Read the model definition and answer for the solid it produces. Units are mm, in the model's axes. Give positions to 0.01 mm unless a question says otherwise; leave off trailing zeros.
```python
from build123d import *

# Parameters (mm, degrees)
SKETCH1_W           = 476.25
SKETCH1_H           = 114.3
BOSS_EXTRUDE1_DEPTH = 6.35
SKETCH2_W           = 463.55
SKETCH2_H           = 6.35
CUT_EXTRUDE1_DEPTH  = 3.175
SKETCH2_3_W         = 463.55
SKETCH2_3_H         = 6.35
SKETCH2_3_W_2       = 469.9
SKETCH2_3_H_2       = 1.5875
CUT_EXTRUDE2_DEPTH  = 3.175


with BuildPart() as part:
    # Sketch1 → Boss-Extrude1 (new body)
    with BuildSketch(Plane(origin=(0, 0, 0), x_dir=(1, 0, 0), z_dir=(0, 1, 0))):
        with Locations((238.125, 57.15)):
            Rectangle(SKETCH1_W, SKETCH1_H)
    extrude(amount=-BOSS_EXTRUDE1_DEPTH)

    # Sketch2 → Cut-Extrude1 (cut)
    with BuildSketch(Plane(origin=(0, 0, 0), x_dir=(1, 0, 0), z_dir=(0, 1, 0))):
        with Locations((238.125, 109.855)):
            Rectangle(SKETCH2_W, SKETCH2_H)
        with BuildLine():
            ThreePointArc((6.35, 106.68), (3.175, 109.855), (6.35, 113.03))
            Line((6.35, 113.03), (6.35, 106.68))
        make_face()
        with Locations((238.125, 56.8325)):
            Rectangle(SKETCH2_W, SKETCH2_H)
        with BuildLine():
            ThreePointArc((6.35, 53.6575), (3.175, 56.8325), (6.35, 60.0075))
            Line((6.35, 60.0075), (6.35, 53.6575))
        make_face()
        with Locations((238.125, 37.7825)):
            Rectangle(SKETCH2_W, SKETCH2_H)
        with BuildLine():
            ThreePointArc((6.35, 34.6075), (3.175, 37.7825), (6.35, 40.9575))
            Line((6.35, 40.9575), (6.35, 34.6075))
        make_face()
        with BuildLine():
            ThreePointArc((6.35, 15.5575), (3.175, 18.7325), (6.35, 21.9075))
            Line((6.35, 21.9075), (6.35, 15.5575))
        make_face()
        with BuildLine():
            ThreePointArc((3.175, 1.27), (2.38125, 2.06375), (3.175, 2.8575))
            Line((3.175, 2.8575), (3.175, 1.27))
        make_face()
        with BuildLine():
            Line((469.9, 106.68), (469.9, 113.03))
            ThreePointArc((469.9, 113.03), (473.075, 109.855), (469.9, 106.68))
        make_face()
        with BuildLine():
            ThreePointArc((469.9, 60.0075), (473.075, 56.8325), (469.9, 53.6575))
            Line((469.9, 53.6575), (469.9, 60.0075))
        make_face()
        with BuildLine():
            ThreePointArc((469.9, 40.9575), (473.075, 37.7825), (469.9, 34.6075))
            Line((469.9, 34.6075), (469.9, 40.9575))
        make_face()
        with BuildLine():
            ThreePointArc((469.9, 21.9075), (473.075, 18.7325), (469.9, 15.5575))
            Line((469.9, 15.5575), (469.9, 21.9075))
        make_face()
        with BuildLine():
            ThreePointArc((473.075, 2.8575), (473.86875, 2.06375), (473.075, 1.27))
            Line((473.075, 1.27), (473.075, 2.8575))
        make_face()
    extrude(amount=-CUT_EXTRUDE1_DEPTH, mode=Mode.SUBTRACT)

    # Sketch2_3 → Cut-Extrude2 (cut)
    with BuildSketch(Plane(origin=(0, 0, 0), x_dir=(1, 0, 0), z_dir=(0, 1, 0))):
        with Locations((238.125, 18.7325)):
            Rectangle(SKETCH2_3_W, SKETCH2_3_H)
        with Locations((238.125, 2.06375)):
            Rectangle(SKETCH2_3_W_2, SKETCH2_3_H_2)
    extrude(amount=-CUT_EXTRUDE2_DEPTH, mode=Mode.SUBTRACT)


solid = part.part
```
1) The part is cut by section A-A on y = -1. Count the separate pieces of the cut face and the enclosed holes in it, and give its area (3 significant figures).
Final values:
separate pieces: 1
enclosed holes: 5
area: 41,800 mm2
2) Given pin 1 (3 mm diameter, centred on x = 151, z = -17.5, fed in from +Y) (3 decimals); pin 2 (1 mm diameter, centred on y = -2, z = -88.5, fed in from -X), each flat-ended and moving along its own axis, determine where each tip first touches the part or whether it passes through.
Final values:
pin 1: stops at y = -3.175
pin 2: stops at x = 0
3) Consider L1, parallel to Z at x = 246, y = -2.75; L2, parallel to X at y = -1, z = -16; L3, parallel to X at y = -1.5, z = -40. Determine where each line is inside the solid, lowest interval first.
Final values:
L1: z = -114.3 to -113.03, -106.68 to -60.01, -53.66 to -40.96, -34.61 to -21.91, -15.56 to -2.86, -1.27 to 0
L2: x = 0 to 4.73, 471.52 to 476.25
L3: x = 0 to 4.08, 472.17 to 476.25
